Read the model definition and answer for the solid it produces. Units are mm, in the model's axes. A direction names the side the tool comes from. Round coordinates to 2 decimals unless told otherwise and drop trailing zeros. Order: outer loops, then holes, each group sorted by start corner. A loop starts at its lowest first (then second) coordinate and runs counter-clockwise, first axis right, second up. Notation, with made-up numbers: (30, -34) - (78, -34) arc R28 ccw to (78, 1) - close; hole circle Ø6 at (2, -37.5). An arc over 180 degrees is marked (long way). One line per question, with ' | ' between items. Start each with the question number.
1) The part is cut by section B-B, the plane y = -0.25. Give the vertices of the cut face in (x, z).
2) Straight lines are drawn through the part: line 1 (Y direction, x = -6, z = 3.25); line 2 (X direction, y = -4.5, z = 20.5); line 3 (X direction, y = 7.3, z = 26). For each, find the intervals that lie inside material, in ascending order. Write a range as from..to.
3) For faces 5 (the flat face through (0, 10, 16)), 6 (the flat face through (0, 6, 18)), determine the directions among +Z, -Z, +X, -X, +Y, -Y from which every point of the face is accessible in a straight line to the end or side of a thin tool.
4) The part is cut by section C-C, the plane x = -1.5. Give the vertices of the cut face in (y, z), plus the area to 3 significant figures.
5) The part is cut by section A-A, the plane z = 26. Give the vertices of the cut face in (x, y), plus the area to 3 significant figures.
6) Flat-ended cylindrical pins translate along their axes: pin 1 (4 mm diameter, centred on x = 6, y = -0.25, fed in from +Z); pin 2 (3.5 mm diameter, centred on x = 2, z = 18.5, fed in from -Y); pin 3 (5 mm diameter, centred on x = -4.5, y = -1, fed in from -Z). Find the tip coordinate at first contact, or state that the pin passes through.
7) The part is cut by section D-D, the plane z = 3. Give the vertices of the cut face in (x, y), plus the area to 3 significant figures.
8) The mould has two halves that part along X. Classify faces 1 (the cylindrical face through (4.81, -1.16, 2.03)), 2 (the flat face through (12, 0, 16)), 3 (the flat face through (-12, 0, 16)), 4 (the flat face through (0, 0, 0)): pulls with the +X half, pulls with the -X half, needs draft (parallel to the pull), parting line crosses it, or undercut.
from build123d import *

# Parameters (mm, degrees)
SKETCH_1_W          = 18
SKETCH_1_H          = 20
EXTRUDE_1_DEPTH     = 4
SKETCH_2_W          = 18
SKETCH_2_H          = 4
EXTRUDE_2_DEPTH     = 28
SKETCH_3_R          = 2.5
CUT_EXTRUDE_1_DEPTH = 37.891733491
SKETCH_4_R          = 1.5
CUT_EXTRUDE_2_DEPTH = 32
EXTRUDE_3_DEPTH     = 3
EXTRUDE_4_DEPTH     = 3
EXTRUDE_5_DEPTH     = 3
EXTRUDE_6_DEPTH     = 3
FILLET_1_R          = 3


with BuildPart() as part:
    # 草图1 → 凸台-拉伸1 (new body)
    with BuildSketch(Plane.XY):
        Rectangle(SKETCH_1_W, SKETCH_1_H)
    extrude(amount=EXTRUDE_1_DEPTH)

    # 草图2 → 凸台-拉伸2 (add)
    with BuildSketch(Plane.XY.offset(4)):
        with Locations((0, 8)):
            Rectangle(SKETCH_2_W, SKETCH_2_H)
    extrude(amount=EXTRUDE_2_DEPTH)

    # 草图3 → 切除-拉伸1 (cut, through all)
    with BuildSketch(Plane.XZ.offset(-6)):
        with Locations(Location((0, 26, 0), (0, 0, 270))):
            Circle(SKETCH_3_R)
    extrude(amount=-CUT_EXTRUDE_1_DEPTH, mode=Mode.SUBTRACT)

    # 草图4 → 切除-拉伸2 (cut)
    with BuildSketch(Plane.XY.offset(4)):
        with Locations((-6, -0.25)):
            Circle(SKETCH_4_R)
        with Locations((-6, -6.75)):
            Circle(SKETCH_4_R)
        with Locations((6, -0.25)):
            Circle(SKETCH_4_R)
        with Locations((6, -6.75)):
            Circle(SKETCH_4_R)
    extrude(amount=-CUT_EXTRUDE_2_DEPTH, mode=Mode.SUBTRACT)

    # 草图5 → 凸台-拉伸3 (add)
    with BuildSketch(Plane(origin=(9, 0, 0), x_dir=(0, 0, -1), z_dir=(1, 0, 0))):
        Polygon((-32, 10), (0, 10), (0, -10), (-4, -10), (-32, 6), align=None)
    extrude(amount=EXTRUDE_3_DEPTH)

    # 草图6 → 凸台-拉伸4 (add)
    with BuildSketch(Plane.ZY.offset(9)):
        Polygon((0, -10), (0, 10), (32, 10), (32, 6), (4, -10), align=None)
    extrude(amount=EXTRUDE_4_DEPTH)

    # 草图7 → 凸台-拉伸5 (add)
    with BuildSketch(Plane.ZY.offset(12)):
        Polygon((32, 6), (4, -10), (32, -10), align=None)
    extrude(amount=-EXTRUDE_5_DEPTH)

    # 草图8 → 凸台-拉伸6 (add)
    with BuildSketch(Plane(origin=(12, 0, 0), x_dir=(0, 0, -1), z_dir=(1, 0, 0))):
        Polygon((-32, 6), (-4, -10), (-32, -10), align=None)
    extrude(amount=-EXTRUDE_6_DEPTH)

    # 圆角1
    fillet_1_edges = [part.edges().sort_by_distance(p)[0] for p in [
        (-9, 6, 18),
        (9, 6, 18),
    ]]
    fillet(fillet_1_edges, radius=FILLET_1_R)


solid = part.part
Values:
1) outline: (-12, 0) - (-7.5, 0) - (-7.5, 4) - (-9, 4) - (-9, 32) - (-12, 32) - close; (-4.5, 0) - (4.5, 0) - (4.5, 4) - (-4.5, 4) - close; (7.5, 0) - (12, 0) - (12, 32) - (9, 32) - (9, 4) - (7.5, 4) - close
2) line 1: y = -10..-8.25, -5.25..-1.75, 1.25..10 | line 2: x = -12..-9, 9..12 | line 3: x = -12..-2.5, 2.5..12
3) face 5: +Z, -Z, +X, -X, +Y | face 6: +Z, -Y
4) outline: (-10, 0) - (10, 0) - (10, 24) - (6, 24) - (6, 4) - (-10, 4) - close; (6, 28) - (10, 28) - (10, 32) - (6, 32) - close | area: 176 mm^2
5) outline: (-12, -10) - (-9, -10) - (-9, 3) arc R3 cw to (-6, 6) - (-2.5, 6) - (-2.5, 10) - (-12, 10) - close; (2.5, 6) - (6, 6) arc R3 cw to (9, 3) - (9, -10) - (12, -10) - (12, 10) - (2.5, 10) - close | area: 176 mm^2
6) pin 1: stops at z = 4 | pin 2: stops at y = 6 | pin 3: stops at z = 0
7) outline: (-12, -10) - (12, -10) - (12, 10) - (-12, 10) - close; hole circle Ø3 at (-6, -6.75); hole circle Ø3 at (-6, -0.25); hole circle Ø3 at (6, -6.75); hole circle Ø3 at (6, -0.25) | area: 452 mm^2
8) face 1: undercut | face 2: pulls with the +X half | face 3: pulls with the -X half | face 4: needs draft
